Check sheet for the modelled part. Datum: model origin and axes. Units: mm. Coordinates: 2 decimals unless noted, no trailing zeros. Write each loop counter-clockwise with the first axis right and the second up, starting at its lowest first coordinate (ties: lowest second). Pieces come first, ordered by that corner, then holes. Notation, with made-up numbers: (75, 86.25) -> (109, 86.25) arc R26 cw to (109, 113.25) -> close; hole circle Ø3 at (83, 7.5). An arc over 180 degrees is marked (long way). One line per item, written item: value. Start each with the question number.
1) Gauge pin test, flat ends, axial feed: P1, Ø11.5, axis at x = 20, y = 0, coming from the +Z side; P2, Ø6, axis at x = -20, y = 0, coming from the -Z side. Record the tip position at first contact, or that the pin passes through.
2) Sectioned sample at B-B on y = 0. Enter the section's corners in (x, z).
3) Scan lines: line 1 along X through (y, z) = (0, 2.5); line 2 along Y through (x, z) = (20, 5); line 3 along X through (y, z) = (-3.75, 4.75). Record each from-to range of solid material in increasing order. Write a range as [from, to].
4) Sectioned sample at D-D on x = 24. Enter the section's corners in (y, z), plus the area to 3 significant figures.
5) Draft check along Y on faces 1 (the cylindrical face through (-24.81, -1.51, 5.07)), 2 (the flat face through (0, 12.5, 5)), 3 (the flat face through (0, -12.5, 5)), 4 (the flat face through (0, 0, 0)). Enter one of: +Y half, -Y half, draft (parallel to the pull), parting line (faces both ways), or undercut.
6) Sectioned sample at A-A on x = -20. Enter the section's corners in (y, z).
7) Sectioned sample at C-C on z = 2.5. Enter the section's corners in (x, y).
```python
from build123d import *

# Parameters (mm, degrees)
F0_W     = 60
F0_H     = 10
F1_DEPTH = 12.5
F2_W     = 5.0413812651
F2_H     = 12


# Not quite as in the source:
# - a pattern or mirror of a feature is missing from the dataset's text; its kind, count and spacing are read off the source's solid


with BuildPart() as f1:
    # F0 (on Front) → F1 (new body, symmetric)
    with BuildSketch(Plane.XZ):
        with Locations((0, 5)):
            Rectangle(F0_W, F0_H)
    extrude(amount=F1_DEPTH, both=True)

    # F2 (on Front) → F3 (revolve, cut)
    with BuildSketch(Plane.XZ):
        with Locations((-22.5206906326, 6)):
            Rectangle(F2_W, F2_H)
    f3 = revolve(axis=Axis((-20, 0, 6), (0, 0, 1)), mode=Mode.SUBTRACT)

    # F3_copies: F3 across plane
    add(f3.mirror(Plane(origin=(0, 0, 0), x_dir=(0, 0, 1), z_dir=(1, 0, 0))), mode=Mode.SUBTRACT)


solid = f1.part
```
Answers:
1. P1: stops at z = 10
1. P2: passes through
2. outline: (-30, 0) -> (-25.04, 0) -> (-25.04, 10) -> (-30, 10) -> close; (-14.96, 0) -> (14.96, 0) -> (14.96, 10) -> (-14.96, 10) -> close; (25.04, 0) -> (30, 0) -> (30, 10) -> (25.04, 10) -> close
3. line 1: x = [-30, -25.04], [-14.96, 14.96], [25.04, 30]
3. line 2: y = [-12.5, -5.04], [5.04, 12.5]
3. line 3: x = [-30, -23.37], [-16.63, 16.63], [23.37, 30]
4. outline: (-12.5, 0) -> (-3.07, 0) -> (-3.07, 10) -> (-12.5, 10) -> close; (3.07, 0) -> (12.5, 0) -> (12.5, 10) -> (3.07, 10) -> close
4. area: 189 mm2
5. face 1: undercut
5. face 2: +Y half
5. face 3: -Y half
5. face 4: draft
6. outline: (-12.5, 0) -> (-5.04, 0) -> (-5.04, 10) -> (-12.5, 10) -> close; (5.04, 0) -> (12.5, 0) -> (12.5, 10) -> (5.04, 10) -> close
7. outline: (-30, -12.5) -> (30, -12.5) -> (30, 12.5) -> (-30, 12.5) -> close; hole circle Ø10.08 at (-20, 0); hole circle Ø10.08 at (20, 0)
